Design review of the part built by this model. Coordinates are the model's own, in mm. Coordinates: 2 decimals unless noted, no trailing zeros. Write each loop counter-clockwise with the first axis right and the second up, starting at its lowest first coordinate (ties: lowest second). Pieces come first, ordered by that corner, then holes. Notation, with made-up numbers: (-9.75, 33) - (5.25, 33) arc R14 cw to (5.25, 59) - close; hole circle Ø3 at (-16, 82). An arc over 180 degrees is marked (long way). Answer as CSV lines item,"result". Start each with the question number.
Q1. We need section B-B (y = 7). Write out the cut boundary in (x, z) (3 decimals).
Q2. We need section C-C (z = 0.85). State how many separate pieces and enclosed holes the cut face has, plus the area to 3 significant figures.
Q3. For line 1 along X through (y, z) = (0.5, 3.05); line 2 along Y through (x, z) = (8, 2.5); line 3 along Y through (x, z) = (-17, 0.3), list the stretches that pass through material, from the lowest coordinate up. Write a range as [from, to].
Q4. We need section A-A (x = 0). Write out the cut boundary in (y, z) (3 decimals), plus the area to 3 significant figures.
Q5. Clearance check with flat-ended pins moving along their axes: pin 1 (5.5 mm diameter, centred on x = 15.22, y = 28.44, fed in from -Z); pin 2 (1.5 mm diameter, centred on y = 10.5, z = 2.5, fed in from -X). State where each tip first meets the part, or that it passes through.
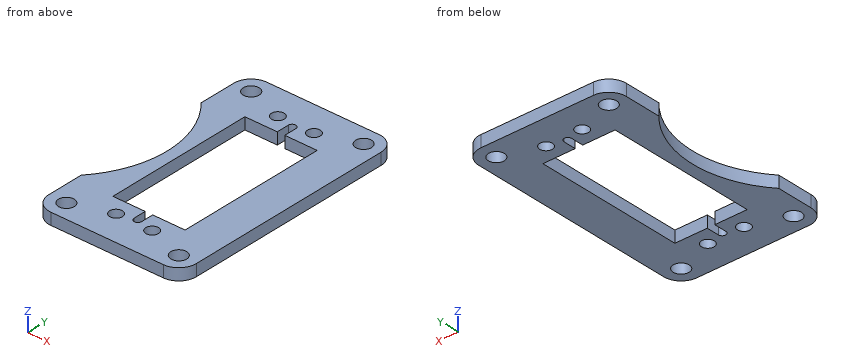
from build123d import *

# Parameters (mm, degrees)
F0_W     = 39.961066
F0_H     = 66.41153
F0_R     = 2.15265
F0_R_2   = 1.7272
F1_DEPTH = 3.175
F2_R     = 4.7625
F4_DEPTH = 3.175


with BuildPart() as f1:
    # F0 (on Top) → F1 (new body)
    with BuildSketch(Plane.XY):
        Rectangle(F0_W, F0_H)
        with Locations((-15.218033, -28.443265)):
            Circle(F0_R, mode=Mode.SUBTRACT)
        with Locations((-4.8895, -24.892)):
            Circle(F0_R_2, mode=Mode.SUBTRACT)
        with Locations((4.8895, -24.892)):
            Circle(F0_R_2, mode=Mode.SUBTRACT)
        with Locations((15.218033, -28.443265)):
            Circle(F0_R, mode=Mode.SUBTRACT)
        with Locations((-15.218033, 28.443265)):
            Circle(F0_R, mode=Mode.SUBTRACT)
        with Locations((-4.8895, 24.892)):
            Circle(F0_R_2, mode=Mode.SUBTRACT)
        with BuildLine():
            Line((-1.016, -20.32), (-9.779, -20.32))
            Line((-9.779, -20.32), (-9.779, 20.32))
            Line((-9.779, 20.32), (-1.016, 20.32))
            Line((-1.016, 20.32), (-1.016, 23.749))
            ThreePointArc((-1.016, 23.749), (0, 24.765), (1.016, 23.749))
            Line((1.016, 23.749), (1.016, 20.32))
            Line((1.016, 20.32), (9.779, 20.32))
            Line((9.779, 20.32), (9.779, -20.32))
            Line((9.779, -20.32), (1.016, -20.32))
            Line((1.016, -20.32), (1.016, -23.749))
            ThreePointArc((1.016, -23.749), (0, -24.765), (-1.016, -23.749))
            Line((-1.016, -23.749), (-1.016, -20.32))
        make_face(mode=Mode.SUBTRACT)
        with Locations((4.8895, 24.892)):
            Circle(F0_R_2, mode=Mode.SUBTRACT)
        with Locations((15.218033, 28.443265)):
            Circle(F0_R, mode=Mode.SUBTRACT)
    extrude(amount=F1_DEPTH)

    # F2
    f2_edges = [f1.edges().sort_by_distance(p)[0] for p in [
        (19.980533, 33.205765, 1.5875),
        (19.980533, -33.205765, 1.5875),
        (-19.980533, 33.205765, 1.5875),
        (-19.980533, -33.205765, 1.5875),
    ]]
    fillet(f2_edges, radius=F2_R)

    # F3 (on face) → F4 (cut, through all)
    with BuildSketch(Plane(origin=(0, 0, 0), x_dir=(1, 0, 0), z_dir=(0, 0, -1))):
        with BuildLine():
            Line((-19.980533, 18.467257), (-19.980533, -18.467257))
            ThreePointArc((-19.980533, -18.467257), (-12.954, 0), (-19.980533, 18.467257))
        make_face()
    extrude(amount=-F4_DEPTH, mode=Mode.SUBTRACT)


solid = f1.part
Results list:
1,outline,"(-13.85, 0) - (-9.779, 0) - (-9.779, 3.175) - (-13.85, 3.175) - close; (9.779, 0) - (19.981, 0) - (19.981, 3.175) - (9.779, 3.175) - close"
2,separate pieces,"1"
2,enclosed holes,"9"
2,area,"1,550 mm2"
3,line 1,"x = [-12.96, -9.78], [9.78, 19.98]"
3,line 2,"y = [-33.21, -20.32], [20.32, 33.21]"
3,line 3,"y = [-32.86, -29.65], [-27.24, -14.44], [14.44, 27.24], [29.65, 32.86]"
4,outline,"(-33.206, 0) - (-24.765, 0) - (-24.765, 3.175) - (-33.206, 3.175) - close; (24.765, 0) - (33.206, 0) - (33.206, 3.175) - (24.765, 3.175) - close"
4,area,"53.6 mm2"
5,pin 1,"stops at z = 0"
5,pin 2,"stops at x = -15.33"
